Study the drawing (mm; zero at the part's minimum x, y, z) and answer. Round coordinates to 2 decimals unless told otherwise and drop trailing zeros. Write each loop counter-clockwise with the first axis right and the second up, starting at its lowest first coordinate (ties: lowest second). Pieces come first, ordered by that corner, then holes. Notation, with made-up numbers: (-20.5, 21.25) -> (33.5, 21.25) arc R12 ccw to (33.5, 41.25) -> close; hole circle Ø2 at (23.5, 43.25). An arc over 180 degrees is marked (long way). Write each question's results on one line, items separated by ' | '. Start each with the question number.
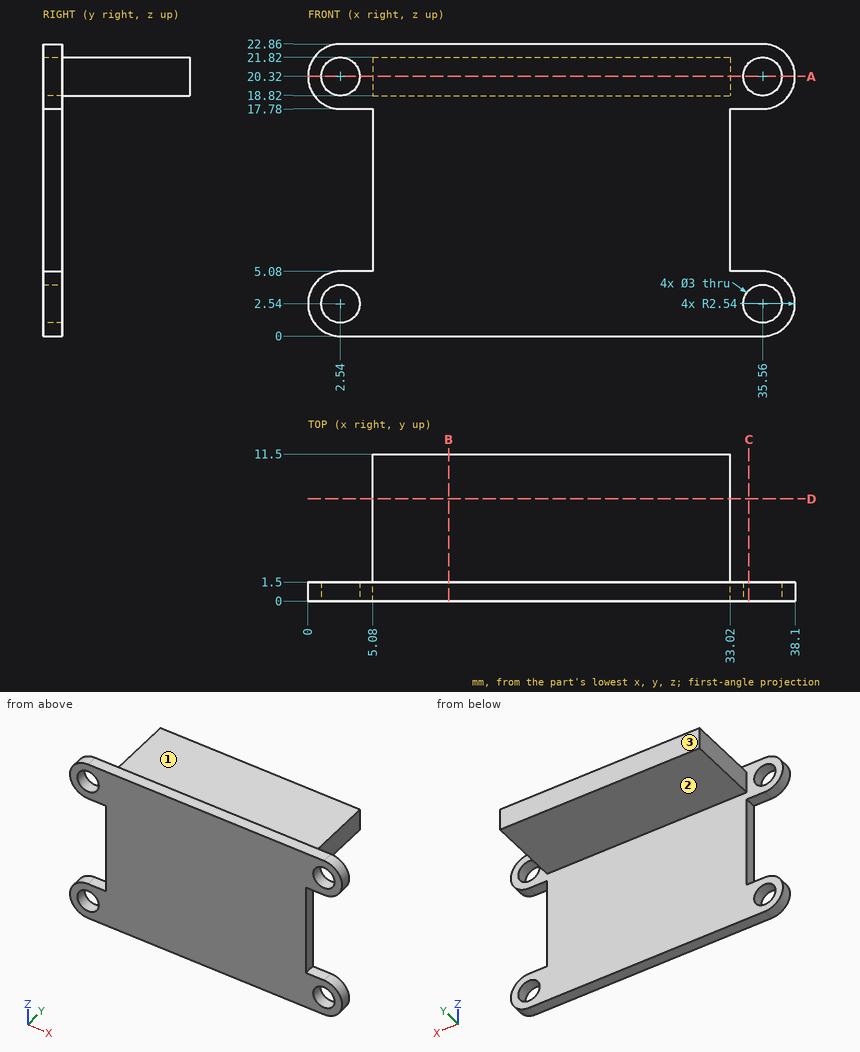
Q1. The part is cut by section A-A, the plane z = 20.32. Write down the section's boundary in (x, y).
Q2. Determine the mould class of the marked faces 1, 2 and 3 for opening direction Z: pulls with the +Z half, pulls with the -Z half, needs draft (parallel to the pull), parting line crosses it, or undercut.
Q3. Find the intervals of material crossed by line 1 (X direction, y = 1, z = 20.32); line 2 (Y direction, x = 9.5, z = 7.25); line 3 (Z direction, x = 24, y = 5.25), in increasing order.
Q4. The part is cut by section D-D, the plane y = 8. Write down the section's boundary in (x, z), then the cut area to 3 significant figures.
Q5. The part is cut by section C-C, the plane x = 34.5. Write down the section's boundary in (y, z).
Q6. Each of these flat-tipped pins is pushed along its axis until it touches: pin 1 (11.5 mm diameter, centred on x = 14, z = 11, fed in from +Y); pin 2 (8 mm diameter, centred on x = 28, z = 9, fed in from -Y); pin 3 (2.5 mm diameter, centred on x = 35.56, z = 2.54, fed in from +Y); pin 4 (0.8 mm diameter, centred on y = 1, z = 9, fed in from -X). Where does it stop, or does it pass through?
Q7. The part is cut by section B-B, the plane x = 11. Write down the section's boundary in (y, z), then the cut area to 3 significant figures.
Answers follow:
1) outline: (0, 0) -> (1.04, 0) -> (1.04, 1.5) -> (0, 1.5) -> close; (4.04, 0) -> (34.06, 0) -> (34.06, 1.5) -> (33.02, 1.5) -> (33.02, 11.5) -> (5.08, 11.5) -> (5.08, 1.5) -> (4.04, 1.5) -> close; (37.06, 0) -> (38.1, 0) -> (38.1, 1.5) -> (37.06, 1.5) -> close
2) face 1: pulls with the +Z half | face 2: pulls with the -Z half | face 3: needs draft
3) line 1: 0 to 1.04, 4.04 to 34.06, 37.06 to 38.1 | line 2: 0 to 1.5 | line 3: 18.82 to 21.82
4) outline: (5.08, 18.82) -> (33.02, 18.82) -> (33.02, 21.82) -> (5.08, 21.82) -> close | area: 83.8 mm^2
5) outline: (0, 0) -> (1.5, 0) -> (1.5, 1.48) -> (0, 1.48) -> close; (0, 3.6) -> (1.5, 3.6) -> (1.5, 5.08) -> (0, 5.08) -> close; (0, 17.78) -> (1.5, 17.78) -> (1.5, 19.26) -> (0, 19.26) -> close; (0, 21.38) -> (1.5, 21.38) -> (1.5, 22.86) -> (0, 22.86) -> close
6) pin 1: y = 1.5 | pin 2: y = 0 | pin 3: through | pin 4: x = 5.08
7) outline: (0, 0) -> (1.5, 0) -> (1.5, 18.82) -> (11.5, 18.82) -> (11.5, 21.82) -> (1.5, 21.82) -> (1.5, 22.86) -> (0, 22.86) -> close | area: 64.3 mm^2
